For this review, take the finished solid that the model builds, in its own axes (mm). A direction names the side the tool comes from. Give positions to 0.01 mm unless a question says otherwise; leave off trailing zeros. Write each loop counter-clockwise with the first axis right and the second up, starting at its lowest first coordinate (ties: lowest second). Pieces come first, ordered by that corner, then holes. Notation, with made-up numbers: (64.25, 15.5) -> (110.25, 15.5) arc R26 ccw to (110.25, 46.5) -> close; hole circle Ø9 at (19, -6.5). An arc over 180 degrees is marked (long way). Return JSON: item names as keys, results as strings.
from build123d import *

# Parameters (mm, degrees)
F1_DEPTH  = 7.5
F2_W      = 8.7
F2_H      = 15
F2_W_2    = 13.2
F3_DEPTH  = 2.2
F4_R      = 2.125
F5_DEPTH  = 25
F7_DEPTH  = 4
F8_R      = 2.125
F9_DEPTH  = 25
F11_DEPTH = 4


with BuildPart() as f1:
    # F0 (on Front) → F1 (new body, symmetric)
    with BuildSketch(Plane.XZ):
        with BuildLine():
            Line((-2.2, 0), (-15.4, 0))
            Line((-15.4, 0), (-15.4, -3.2))
            Line((-15.4, -3.2), (-5.4, -3.2))
            Line((-5.4, -3.2), (-5.4, -13.8))
            ThreePointArc((-5.4, -13.8), (-4.667767, -15.567767), (-2.9, -16.3))
            Line((-2.9, -16.3), (2.3, -16.3))
            ThreePointArc((2.3, -16.3), (4.067767, -15.567767), (4.8, -13.8))
            Line((4.8, -13.8), (4.8, -3.2))
            Line((4.8, -3.2), (20, -3.2))
            Line((20, -3.2), (20, 0))
            Line((20, 0), (0, 0))
            Line((0, 0), (0, -11.3))
            Line((0, -11.3), (-2.2, -11.3))
            Line((-2.2, -11.3), (-2.2, 0))
        make_face()
    extrude(amount=F1_DEPTH, both=True)

    # F2 (on face) → F3 (join)
    with BuildSketch(Plane.XY):
        with Locations((15.65, 0)):
            Rectangle(F2_W, F2_H)
        with Locations((-8.8, 0)):
            Rectangle(F2_W_2, F2_H)
    extrude(amount=F3_DEPTH)

    # F4 (on face) → F5 (cut)
    with BuildSketch(Plane.XY.offset(2.2)):
        with Locations((-10.4, 0)):
            Circle(F4_R)
        with Locations((15, 0)):
            Circle(F4_R)
    extrude(amount=-F5_DEPTH, mode=Mode.SUBTRACT)

    # F6 (on face) → F7 (cut)
    with BuildSketch(Plane(origin=(0, 0, -3.2), x_dir=(1, 0, 0), z_dir=(0, 0, -1))):
        Polygon((-7.475, -1.68875), (-7.475, 1.68875), (-10.4, 3.377499), (-13.325, 1.68875), (-13.325, -1.68875), (-10.4, -3.377499), align=None)
        Polygon((17.925, -1.68875), (17.925, 1.68875), (15, 3.377499), (12.075, 1.68875), (12.075, -1.68875), (15, -3.377499), align=None)
    extrude(amount=-F7_DEPTH, mode=Mode.SUBTRACT)

    # F8 (on face) → F9 (cut)
    with BuildSketch(Plane.YZ.offset(4.8)):
        with Locations((0, -6.35)):
            Circle(F8_R)
    extrude(amount=-F9_DEPTH, mode=Mode.SUBTRACT)

    # F10 (on face) → F11 (cut)
    with BuildSketch(Plane.YZ.offset(4.8)):
        Polygon((-1.68875, -9.275), (1.68875, -9.275), (3.377499, -6.35), (1.68875, -3.425), (-1.68875, -3.425), (-3.377499, -6.35), align=None)
    extrude(amount=-F11_DEPTH, mode=Mode.SUBTRACT)


solid = f1.part
1. Add section A-A, the plane z = -6. State the section outline as (x, y) points, plus the area to 3 significant figures.
Results found:
{"outline": "(-5.4, -7.5) -> (-2.2, -7.5) -> (-2.2, -2.1) -> (-5.4, -2.1) -> close; (-5.4, 2.1) -> (-2.2, 2.1) -> (-2.2, 7.5) -> (-5.4, 7.5) -> close; (0, -7.5) -> (4.8, -7.5) -> (4.8, -3.18) -> (0.8, -3.18) -> (0.8, -2.1) -> (0, -2.1) -> close; (0, 2.1) -> (0.8, 2.1) -> (0.8, 3.18) -> (4.8, 3.18) -> (4.8, 7.5) -> (0, 7.5) -> close", "area": "77.8 mm²"}
2. Add section D-D, the plane y = 0. Count the separate pieces of the cut face and the enclosed holes in it, plus the area to 3 significant figures.
Results found:
{"separate pieces": "5", "enclosed holes": "0", "area": "168 mm²"}
3. Add section C-C, the plane x = 10. State the section outline as (y, z) points.
Results found:
{"outline": "(-7.5, -3.2) -> (7.5, -3.2) -> (7.5, 0) -> (-7.5, 0) -> close"}
4. To check wall thickness, follow probe 1 along X at (y, z) = (5, -7.5); probe 2 along Y at (x, z) = (-10.4, 1.2) (3 decimals); probe 3 along X at (y, z) = (-1.75, -13.5). State the ranges of each line that lie inside material, in increasing order.
Results found:
{"probe 1": "x = -5.4 to -2.2, 0 to 4.8", "probe 2": "y = -7.5 to -2.125, 2.125 to 7.5", "probe 3": "x = -5.4 to 4.8"}
5. The part is to be moulded in two halves that separate along Z. For faces 5 (the flat face through (6, 0, 0)), 6 (the flat face through (2.828, -2.545, -7.792)), 7 (the flat face through (14.3, 2.2, 0.8)), say which applies: +Z half, -Z half, draft (parallel to the pull), parting line (faces both ways), or undercut.
Results found:
{"face 5": "+Z half", "face 6": "undercut", "face 7": "-Z half"}
6. For pin 1 (5 mm diameter, centred on x = -9, y = -0.5, fed in from -Z); pin 2 (0.7 mm diameter, centred on x = -1, y = 3, fed in from +Z); pin 3 (5 mm diameter, centred on y = 5.5, z = -10.5, fed in from -X), all flat-tipped, find the tip position at first contact; note any pin that passes through.
Results found:
{"pin 1": "stops at z = -3.2", "pin 2": "stops at z = -11.3", "pin 3": "stops at x = -5.4"}
7. Add section B-B, the plane y = 6. State the section outline as (x, z) points.
Results found:
{"outline": "(-15.4, -3.2) -> (-5.4, -3.2) -> (-5.4, -13.8) arc R2.5 ccw to (-2.9, -16.3) -> (2.3, -16.3) arc R2.5 ccw to (4.8, -13.8) -> (4.8, -3.2) -> (20, -3.2) -> (20, 2.2) -> (11.3, 2.2) -> (11.3, 0) -> (0, 0) -> (0, -11.3) -> (-2.2, -11.3) -> (-2.2, 2.2) -> (-15.4, 2.2) -> close"}
8. For faces 1 (the flat face through (-2.2, 0, -3)), 2 (the flat face through (2.828, -2.521, -4.867)), 3 (the flat face through (-7, 0, -3.2)), 4 (the flat face through (-8.958, 2.545, -1.228)), list the 3-axis set-ups (+Z, -Z, +X, -X, +Y, -Y) from which the entire face can be reached by the end or side of a thin tool; tool diameter is ignored.
Results found:
{"face 1": "+Z, +Y, -Y", "face 2": "+X", "face 3": "-Z, -X, +Y, -Y", "face 4": "-Z"}
